Check sheet for the modelled part. Datum: model origin and axes. Units: mm. Coordinates: 2 decimals unless noted, no trailing zeros. Answer as CSV lines item,"result". Start each with the question number.
1) Go/stop test with flat-tipped pins: pin 1 Ø0.8 at (x, z) = (-1.5, 257) entering from +Y; pin 2 Ø2 at (y, z) = (-21.5, 182) entering from +X; pin 3 Ø1.3 at (y, z) = (-1.5, 327) entering from -X. Record where each tip stops, or that it passes through.
2) Section check A-A (z = 36). State how many separate pieces and enclosed holes the cut face has, and give its area (3 significant figures).
3) Material ranges on L1, parallel to Y at x = -7.25, z = 96; L2, parallel to Y at x = 0, z = 333; L3, parallel to X at y = 4.5, z = 266, recorded low to high. Write a range as [from, to].
from build123d import *
from build123d.topology import SkipClean

# Parameters (mm, degrees)
BOSS_EXTRU_1_DEPTH     = 560.3
SYM_TRIE6_COPY_1_DEPTH = 560.3


with BuildPart() as part:
    # Esquisse1 → Boss.-Extru.1 (new body)
    with BuildSketch(Plane.XY):
        with BuildLine():
            Line((-9.5, 10), (-4.58, 10))
            Line((-4.58, 10), (-3.125, 8.545))
            Line((-3.125, 8.545), (-3.125, 8.2))
            Line((-3.125, 8.2), (-5.5, 8.2))
            Line((-5.5, 8.2), (-5.5, 6.560660172))
            Line((-5.5, 6.560660172), (-2.839339828, 3.9))
            Line((-2.839339828, 3.9), (-0.21, 3.9))
            Line((-0.21, 3.9), (0, 3.69))
            Line((0, 3.69), (0, 2.1))
            ThreePointArc((0, 2.1), (-2.1, 0), (0, -2.1))
            Line((0, -2.1), (0, -3.69))
            Line((0, -3.69), (-0.21, -3.9))
            Line((-0.21, -3.9), (-2.839339828, -3.9))
            Line((-2.839339828, -3.9), (-6.239339828, -7.3))
            Line((-6.239339828, -7.3), (-8.2, -7.3))
            Line((-8.2, -7.3), (-8.2, -10))
            Line((-8.2, -10), (-10, -10))
            Line((-10, -10), (-10, -4.58))
            Line((-10, -4.58), (-8.545, -3.125))
            Line((-8.545, -3.125), (-8.2, -3.125))
            Line((-8.2, -3.125), (-8.2, -5.5))
            Line((-8.2, -5.5), (-6.560660172, -5.5))
            Line((-6.560660172, -5.5), (-3.9, -2.839339828))
            Line((-3.9, -2.839339828), (-3.9, -0.21))
            Line((-3.9, -0.21), (-3.69, 0))
            Line((-3.69, 0), (-3.9, 0.21))
            Line((-3.9, 0.21), (-3.9, 2.839339828))
            Line((-3.9, 2.839339828), (-6.560660172, 5.5))
            Line((-6.560660172, 5.5), (-8.2, 5.5))
            Line((-8.2, 5.5), (-8.2, 3.125))
            Line((-8.2, 3.125), (-8.545, 3.125))
            Line((-8.545, 3.125), (-10, 4.58))
            Line((-10, 4.58), (-10, 9.5))
            ThreePointArc((-10, 9.5), (-9.853553391, 9.853553391), (-9.5, 10))
        make_face()
    boss_extru_1 = extrude(amount=BOSS_EXTRU_1_DEPTH)

    # Symétrie1: Boss.-Extru.1 across plane
    add(boss_extru_1.mirror(Plane(origin=(0, 3.69, 560.3), x_dir=(0, 0, 1), z_dir=(-1, 0, 0))))

    # Symétrie6: Boss.-Extru.1 across plane
    add(boss_extru_1.mirror(Plane(origin=(-8.2, -10, 560.3), x_dir=(0, 0, 1), z_dir=(0, 1, 0))))

    # Symétrie6 copy 1 sketch → Symétrie6 copy 1 (add)
    with SkipClean():  # the faces are left unmerged after this step: merging them gives an invalid solid
        with BuildSketch(Plane(origin=(0, -20, 0), x_dir=(-1, 0, 0), z_dir=(0, 0, 1))):
            with BuildLine():
                Line((-9.5, 10), (-4.58, 10))
                Line((-4.58, 10), (-3.125, 8.545))
                Line((-3.125, 8.545), (-3.125, 8.2))
                Line((-3.125, 8.2), (-5.5, 8.2))
                Line((-5.5, 8.2), (-5.5, 6.560660172))
                Line((-5.5, 6.560660172), (-2.839339828, 3.9))
                Line((-2.839339828, 3.9), (-0.21, 3.9))
                Line((-0.21, 3.9), (0, 3.69))
                Line((0, 3.69), (0, 2.1))
                ThreePointArc((0, 2.1), (-2.1, 0), (0, -2.1))
                Line((0, -2.1), (0, -3.69))
                Line((0, -3.69), (-0.21, -3.9))
                Line((-0.21, -3.9), (-2.839339828, -3.9))
                Line((-2.839339828, -3.9), (-6.239339828, -7.3))
                Line((-6.239339828, -7.3), (-8.2, -7.3))
                Line((-8.2, -7.3), (-8.2, -10))
                Line((-8.2, -10), (-10, -10))
                Line((-10, -10), (-10, -4.58))
                Line((-10, -4.58), (-8.545, -3.125))
                Line((-8.545, -3.125), (-8.2, -3.125))
                Line((-8.2, -3.125), (-8.2, -5.5))
                Line((-8.2, -5.5), (-6.560660172, -5.5))
                Line((-6.560660172, -5.5), (-3.9, -2.839339828))
                Line((-3.9, -2.839339828), (-3.9, -0.21))
                Line((-3.9, -0.21), (-3.69, 0))
                Line((-3.69, 0), (-3.9, 0.21))
                Line((-3.9, 0.21), (-3.9, 2.839339828))
                Line((-3.9, 2.839339828), (-6.560660172, 5.5))
                Line((-6.560660172, 5.5), (-8.2, 5.5))
                Line((-8.2, 5.5), (-8.2, 3.125))
                Line((-8.2, 3.125), (-8.545, 3.125))
                Line((-8.545, 3.125), (-10, 4.58))
                Line((-10, 4.58), (-10, 9.5))
                ThreePointArc((-10, 9.5), (-9.853553391, 9.853553391), (-9.5, 10))
            make_face()
        extrude(amount=SYM_TRIE6_COPY_1_DEPTH)


solid = part.part
Results found:
1,pin 1,"stops at y = 3.9"
1,pin 2,"stops at x = 3.9"
1,pin 3,"stops at x = -3.9"
2,separate pieces,"1"
2,enclosed holes,"3"
2,area,"300 mm2"
3,L1,"y = [-30, -25.5], [-14.5, -12.7], [-7.3, -5.5], [5.5, 10]"
3,L2,"y = [-23.69, -22.1], [-17.9, -16.31], [-3.69, -2.1], [2.1, 3.69]"
3,L3,"x = [-9.92, -8.2], [-5.56, -3.44], [3.44, 5.56], [8.2, 9.92]"
